from build123d import *

# Parameters (mm, degrees)
S_CYL1_R     = 9.8
BOSS_1_DEPTH = 0.4
S_HOLE2_R    = 3.5
HOLE_2_DEPTH = 0.6
S_HOLE3_R    = 1.7
HOLE_3_DEPTH = 0.6
S_HOLE4_R    = 1.7
HOLE_4_DEPTH = 0.6
S_HOLE5_R    = 1.7
HOLE_5_DEPTH = 0.6
S_HOLE6_R    = 1.7
HOLE_6_DEPTH = 0.6


with BuildPart() as part:
    # S_cyl1 → Boss_1 (new body)
    with BuildSketch(Plane.XY):
        Circle(S_CYL1_R)
    extrude(amount=BOSS_1_DEPTH)

    # S_hole2 → Hole_2 (cut)
    with BuildSketch(Plane.XY.offset(-0.1)):
        Circle(S_HOLE2_R)
    extrude(amount=HOLE_2_DEPTH, mode=Mode.SUBTRACT)

    # S_hole3 → Hole_3 (cut)
    with BuildSketch(Plane.XY.offset(-0.1)):
        with Locations((7, 0)):
            Circle(S_HOLE3_R)
    extrude(amount=HOLE_3_DEPTH, mode=Mode.SUBTRACT)

    # S_hole4 → Hole_4 (cut)
    with BuildSketch(Plane.XY.offset(-0.1)):
        with Locations((0, 7)):
            Circle(S_HOLE4_R)
    extrude(amount=HOLE_4_DEPTH, mode=Mode.SUBTRACT)

    # S_hole5 → Hole_5 (cut)
    with BuildSketch(Plane.XY.offset(-0.1)):
        with Locations((-7, 0)):
            Circle(S_HOLE5_R)
    extrude(amount=HOLE_5_DEPTH, mode=Mode.SUBTRACT)

    # S_hole6 → Hole_6 (cut)
    with BuildSketch(Plane.XY.offset(-0.1)):
        with Locations((0, -7)):
            Circle(S_HOLE6_R)
    extrude(amount=HOLE_6_DEPTH, mode=Mode.SUBTRACT)


solid = part.part
Check sheet for the modelled part. Datum: model origin and axes. Units: mm. Round coordinates to 2 decimals unless told otherwise and drop trailing zeros. Order: outer loops, then holes, each group sorted by start corner. A loop starts at its lowest first (then second) coordinate and runs counter-clockwise, first axis right, second up.
(1) Cross-section at A-A, the plane y = 0. Enter the section's corners in (x, z), and give its area (3 significant figures).
(2) Cross-section at B-B, the plane x = -1. Enter the section's corners in (y, z).
(3) Scan lines: probe 1 along Y at (x, z) = (0, 0.3); probe 2 along Y at (x, z) = (0.5, 0.1); probe 3 along X at (y, z) = (0.25, 0.1). Record each from-to range of solid material in increasing order.
(4) Go/stop test with flat-tipped pins: P1, Ø4, axis at x = 7.5, y = -1.5, coming from the +Z side; P2, Ø3, axis at x = 7, y = 0, coming from the -Z side. Record where each tip stops, or that it passes through.
(5) Cross-section at C-C, the plane y = 3.25. Enter the section's corners in (x, z).
(6) Cross-section at D-D, the plane z = 0.1. Enter the section's corners in (x, y).
(7) Draft check along Y on faces 1 (the flat face through (4, 0, 0.4)), 2 (the cylindrical face through (-2.124, -9.567, 0.197)), 3 (the cylindrical face through (3.233, -1.341, 0.197)). Enter one of: pulls with the +Y half, pulls with the -Y half, needs draft (parallel to the pull), parting line crosses it, or undercut.
Check sheet entries:
1. outline: (-9.8, 0) - (-8.7, 0) - (-8.7, 0.4) - (-9.8, 0.4) - close; (-5.3, 0) - (-3.5, 0) - (-3.5, 0.4) - (-5.3, 0.4) - close; (3.5, 0) - (5.3, 0) - (5.3, 0.4) - (3.5, 0.4) - close; (8.7, 0) - (9.8, 0) - (9.8, 0.4) - (8.7, 0.4) - close
1. area: 2.32 mm2
2. outline: (-9.75, 0) - (-8.37, 0) - (-8.37, 0.4) - (-9.75, 0.4) - close; (-5.63, 0) - (-3.35, 0) - (-3.35, 0.4) - (-5.63, 0.4) - close; (3.35, 0) - (5.63, 0) - (5.63, 0.4) - (3.35, 0.4) - close; (8.37, 0) - (9.75, 0) - (9.75, 0.4) - (8.37, 0.4) - close
3. probe 1: y = -9.8 to -8.7, -5.3 to -3.5, 3.5 to 5.3, 8.7 to 9.8
3. probe 2: y = -9.79 to -8.62, -5.38 to -3.46, 3.46 to 5.38, 8.62 to 9.79
3. probe 3: x = -9.8 to -8.68, -5.32 to -3.49, 3.49 to 5.32, 8.68 to 9.8
4. P1: stops at z = 0.4
4. P2: passes through
5. outline: (-9.25, 0) - (-1.3, 0) - (-1.3, 0.4) - (-9.25, 0.4) - close; (1.3, 0) - (9.25, 0) - (9.25, 0.4) - (1.3, 0.4) - close
6. outline: circle Ø19.6 at (0, 0); hole circle Ø3.4 at (-7, 0); hole circle Ø7 at (0, 0); hole circle Ø3.4 at (0, -7); hole circle Ø3.4 at (0, 7); hole circle Ø3.4 at (7, 0)
7. face 1: needs draft
7. face 2: parting line crosses it
7. face 3: undercut
